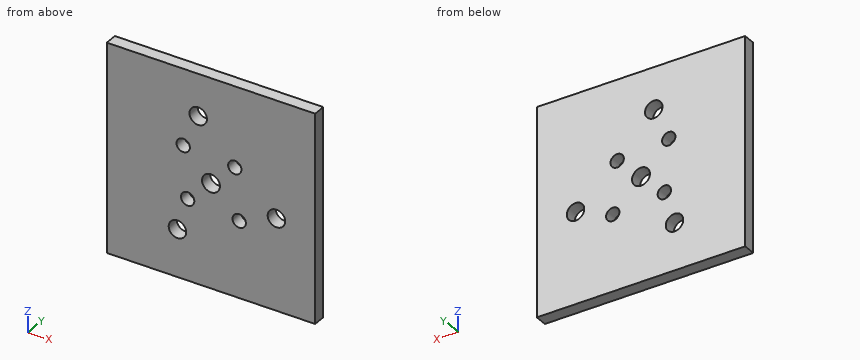
```python
from build123d import *

# Parameters (mm, degrees)
SKETCH1_W           = 50
SKETCH1_H           = 50
BOSS_EXTRUDE1_DEPTH = 3
SKETCH2_R           = 2.15
CUT_EXTRUDE1_DEPTH  = 4
SKETCH3_R           = 1.6
CUT_EXTRUDE2_DEPTH  = 4
SKETCH4_R           = 2.1
CUT_EXTRUDE3_DEPTH  = 4


with BuildPart() as part:
    # Sketch1 → Boss-Extrude1 (new body)
    with BuildSketch(Plane(origin=(0, 0, 0), x_dir=(1, 0, 0), z_dir=(0, 1, 0))):
        Rectangle(SKETCH1_W, SKETCH1_H)
    extrude(amount=-BOSS_EXTRUDE1_DEPTH)

    # Sketch2 → Cut-Extrude1 (cut, through all)
    with BuildSketch(Plane(origin=(0, 0, 0), x_dir=(1, 0, 0), z_dir=(0, 1, 0))):
        Circle(SKETCH2_R)
    extrude(amount=-CUT_EXTRUDE1_DEPTH, mode=Mode.SUBTRACT)

    # Sketch3 → Cut-Extrude2 (cut, through all)
    with BuildSketch(Plane(origin=(0, 0, 0), x_dir=(1, 0, 0), z_dir=(0, 1, 0))):
        with Locations((6.768353811, 6.657078174)):
            Circle(SKETCH3_R)
        with Locations((-6.661646189, -6.772921826)):
            Circle(SKETCH3_R)
        with Locations((-5.601646189, 5.597078174)):
            Circle(SKETCH3_R)
        with Locations((5.708353811, -5.712921826)):
            Circle(SKETCH3_R)
    extrude(amount=-CUT_EXTRUDE2_DEPTH, mode=Mode.SUBTRACT)

    # Sketch4 → Cut-Extrude3 (cut, through all)
    with BuildSketch(Plane(origin=(0, 0, 0), x_dir=(1, 0, 0), z_dir=(0, 1, 0))):
        with Locations((15.70537943, 3.056314275)):
            Circle(SKETCH4_R)
        with Locations((-3.064333665, -14.935291276)):
            Circle(SKETCH4_R)
        with Locations((-8.045828007, 13.633655399)):
            Circle(SKETCH4_R)
    extrude(amount=-CUT_EXTRUDE3_DEPTH, mode=Mode.SUBTRACT)


solid = part.part
```
The listing builds one solid part. Answer for the finished solid, in the listing's coordinates (mm). Coordinates: 2 decimals unless noted, no trailing zeros. Loops run counter-clockwise (first coordinate to the right, second up) from the corner with the lowest first, then second, coordinate; pieces in that order, holes last. Notation, with made-up numbers: (82.5, 44) -> (111.5, 44) arc R14 ccw to (111.5, 68) -> close; hole circle Ø9 at (31, 64). An arc over 180 degrees is marked (long way). Use one line per item in the form item = value. Start each with the question number.
Item 1: The part is cut by section A-A on x = 0. Determine the outline of the cut face in (y, z).
Item 2: Consider L1, parallel to X at y = -1.5, z = 15; L2, parallel to Z at x = 0, y = -2.65; L3, parallel to Z at x = -2.5, y = -1.5. Determine where each line is inside the solid, lowest interval first. Write a range as [from, to].
Item 3: The part is cut by section C-C on y = -1.1. Count the separate pieces of the cut face and the enclosed holes in it, then the cut area to 3 significant figures.
Item 4: The part is cut by section B-B on z = 0. Determine the outline of the cut face in (x, y).
Answer key:
q1.outline = (-3, -25) -> (0, -25) -> (0, -2.15) -> (-3, -2.15) -> close; (-3, 2.15) -> (0, 2.15) -> (0, 25) -> (-3, 25) -> close
q2.L1 = [-25, -5.16], [-0.97, 25]
q2.L2 = [-25, -2.15], [2.15, 25]
q2.L3 = [-25, 12.91], [16.96, 25]
q3.separate_pieces = 1
q3.enclosed_holes = 8
q3.area = 2,410 mm2
q4.outline = (-25, -3) -> (-2.15, -3) -> (-2.15, 0) -> (-25, 0) -> close; (2.15, -3) -> (25, -3) -> (25, 0) -> (2.15, 0) -> close
